Design review of the part built by this model. Coordinates are the model's own, in mm. Face numbers are marked on the shaded views. A direction names the side the tool comes from. Round coordinates to 2 decimals unless told otherwise and drop trailing zeros. Order: outer loops, then holes, each group sorted by start corner. A loop starts at its lowest first (then second) coordinate and runs counter-clockwise, first axis right, second up.
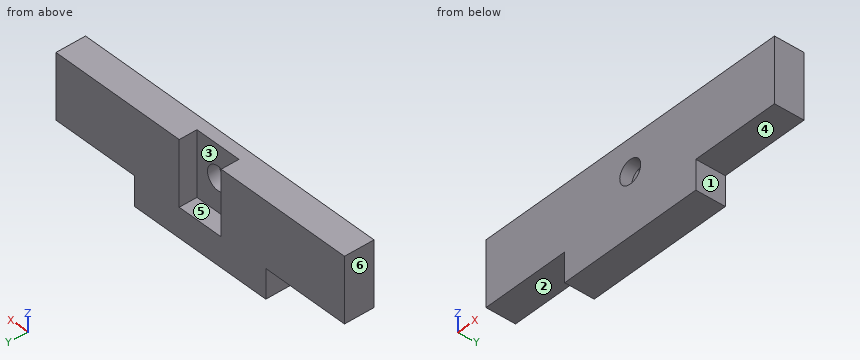
from build123d import *

# Parameters (mm, degrees)
BOSS_EXTRU_1_DEPTH      = 5
ESQUISSE2_W             = 8
ESQUISSE2_H             = 11
ENL_V_MAT_EXTRU_5_DEPTH = 3
ESQUISSE3_R             = 2
ENL_V_MAT_EXTRU_6_DEPTH = 29.7967012


with BuildPart() as part:
    # Esquisse1 → Boss.-Extru.1 (new body)
    with BuildSketch(Plane(origin=(0, 0, 0), x_dir=(1, 0, 0), z_dir=(0, 1, 0))):
        Polygon((-12.5, 8), (-12.5, 3), (-27.5, 3), (-27.5, -8), (27.5, -8), (27.5, 3), (12.5, 3), (12.5, 8), align=None)
    extrude(amount=BOSS_EXTRU_1_DEPTH)

    # Esquisse2 → Enlèv. mat.-Extru.5 (cut)
    with BuildSketch(Plane(origin=(0, 5, 0), x_dir=(1, 0, 0), z_dir=(0, 1, 0))):
        with Locations((0, -2.5)):
            Rectangle(ESQUISSE2_W, ESQUISSE2_H)
    extrude(amount=-ENL_V_MAT_EXTRU_5_DEPTH, mode=Mode.SUBTRACT)

    # Esquisse3 → Enlèv. mat.-Extru.6 (cut, through all)
    with BuildSketch(Plane(origin=(0, 2, 0), x_dir=(1, 0, 0), z_dir=(0, 1, 0))):
        with Locations(Location((0, -2.5, 0), (0, 0, 270))):
            Circle(ESQUISSE3_R)
    extrude(amount=-ENL_V_MAT_EXTRU_6_DEPTH, mode=Mode.SUBTRACT)


solid = part.part
1) Clearance check with flat-ended pins moving along their axes: P1, Ø0.9, axis at x = 0.5, y = 3, coming from the +Z side; P2, Ø2.5, axis at y = 3.5, z = -4.5, coming from the +X side; P3, Ø2.5, axis at x = 19, y = 2.5, coming from the -Z side. State where each tip first meets the part, or that it passes through.
Results:
P1: stops at z = -3
P2: stops at x = 12.5
P3: stops at z = -3
2) Take a section at A-A on z = 2.5. Give the boundary of the cut face in (x, y).
Results:
outline: (-27.5, 0) - (-2, 0) - (-2, 2) - (-4, 2) - (-4, 5) - (-27.5, 5) - close; (2, 0) - (27.5, 0) - (27.5, 5) - (4, 5) - (4, 2) - (2, 2) - close
3) To check wall thickness, follow line 1 along X through (y, z) = (1, 2.5); line 2 along Y through (x, z) = (-2.5, 3.75); line 3 along Z through (x, y) = (22, 3.85). State the ranges of each line that lie inside material, in increasing order.
Results:
line 1: x = -27.5 to -2, 2 to 27.5
line 2: y = 0 to 2
line 3: z = -3 to 8
4) Take a section at C-C on y = 3. Give the boundary of the cut face in (x, z), plus the area to 3 significant figures.
Results:
outline: (-27.5, -3) - (-12.5, -3) - (-12.5, -8) - (12.5, -8) - (12.5, -3) - (27.5, -3) - (27.5, 8) - (4, 8) - (4, -3) - (-4, -3) - (-4, 8) - (-27.5, 8) - close
area: 642 mm2
5) The part is to be moulded in two halves that separate along X. For the marked faces 4, 5 and 6, say which applies: released by +X, released by -X, zero draft, split by the parting line, or undercut.
Results:
face 4: zero draft
face 5: undercut
face 6: released by -X
6) Take a section at B-B on x = 0. Give the boundary of the cut face in (y, z), plus the area to 3 significant figures.
Results:
outline: (0, -8) - (5, -8) - (5, -3) - (2, -3) - (2, 0.5) - (0, 0.5) - close; (0, 4.5) - (2, 4.5) - (2, 8) - (0, 8) - close
area: 39.0 mm2
7) For the marked faces 1, 2 and 3, list the 3-axis set-ups (+Z, -Z, +X, -X, +Y, -Y) from which the entire face can be reached by the end or side of a thin tool; tool diameter is ignored.
Results:
face 1: -Z, +X, +Y, -Y
face 2: -Z, -X, +Y, -Y
face 3: +Z, +Y
8) Take a section at D-D on z = -1. Give the boundary of the cut face in (x, y), plus the area to 3 significant figures.
Results:
outline: (-27.5, 0) - (27.5, 0) - (27.5, 5) - (4, 5) - (4, 2) - (-4, 2) - (-4, 5) - (-27.5, 5) - close
area: 251 mm2
